The drawing under review shows one solid part. Ordinate dimensions are in mm from its lowest x, y, z. Round coordinates to 2 decimals unless told otherwise and drop trailing zeros. Order: outer loops, then holes, each group sorted by start corner. A loop starts at its lowest first (then second) coordinate and runs counter-clockwise, first axis right, second up.
1) Consider section C-C (z = 1.75). Give the boundary of the cut face in (x, y).
2) Consider section B-B (y = 25). Give the boundary of the cut face in (x, z), then the cut area to 3 significant figures.
3) To check wall thickness, follow L1, parallel to Y at x = 16, z = 3; L2, parallel to Y at x = 19.5, z = 6.75; L3, parallel to X at y = 59, z = 4.5. State the ranges of each line that lie inside material, in increasing order.
4) Clearance check with flat-ended pins moving along their axes: P1, Ø1, axis at x = 22.5, y = 40, coming from the -Z side; P2, Ø1.5, axis at x = 10, z = 5, coming from the -Y side. State where each tip first meets the part, or that it passes through.
5) Consider section A-A (x = 16). Give the boundary of the cut face in (y, z), then the cut area to 3 significant figures.
6) Mouldability with a two-part tool opening along Y and no side actions: class the marked faces 1, 2 and 3 as pulls with the +Y half, pulls with the -Y half, needs draft (parallel to the pull), parting line crosses it, or undercut.
7) Consider section D-D (y = 62). Give the boundary of the cut face in (x, z).
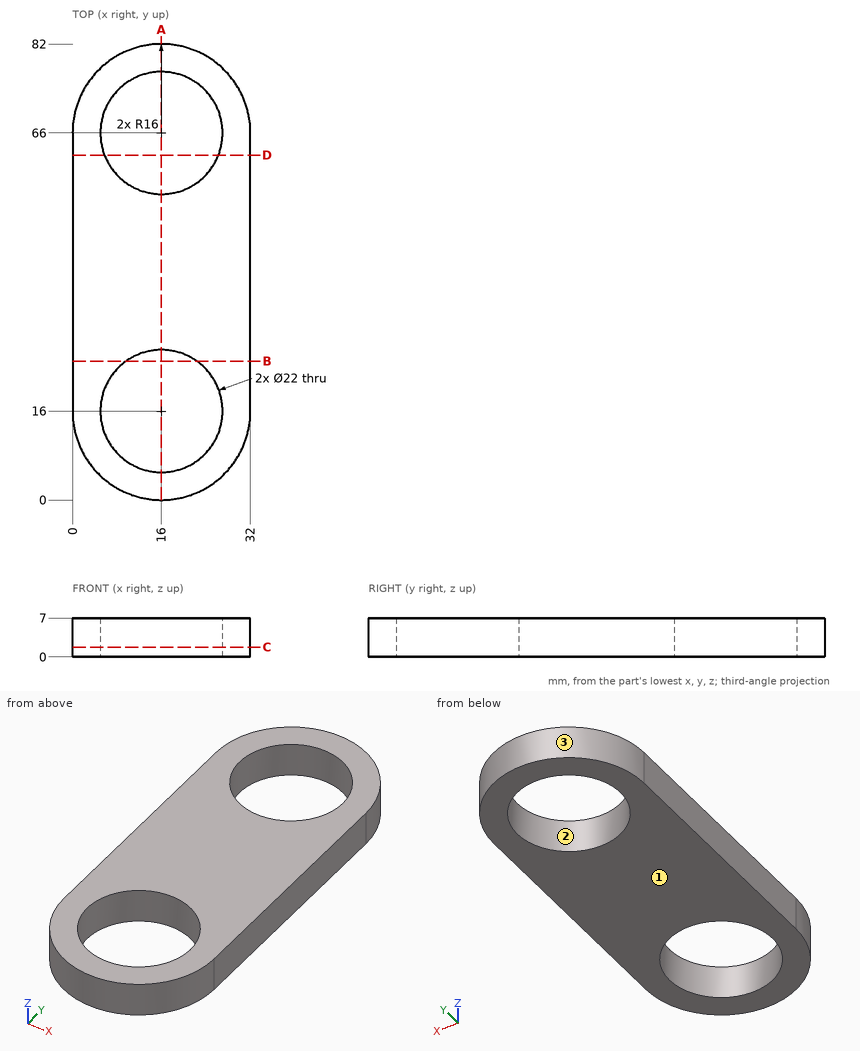
Answer below:
1. outline: (0, 16) arc R16 ccw to (32, 16) - (32, 66) arc R16 ccw to (0, 66) - close; hole circle Ø22 at (16, 16); hole circle Ø22 at (16, 66)
2. outline: (0, 0) - (9.68, 0) - (9.68, 7) - (0, 7) - close; (22.32, 0) - (32, 0) - (32, 7) - (22.32, 7) - close
2. area: 135 mm2
3. L1: y = 0 to 5, 27 to 55, 77 to 82
3. L2: y = 0.39 to 5.57, 26.43 to 55.57, 76.43 to 81.61
3. L3: x = 0 to 7.51, 24.49 to 32
4. P1: stops at z = 0
4. P2: stops at y = 0.89
5. outline: (0, 0) - (5, 0) - (5, 7) - (0, 7) - close; (27, 0) - (55, 0) - (55, 7) - (27, 7) - close; (77, 0) - (82, 0) - (82, 7) - (77, 7) - close
5. area: 266 mm2
6. face 1: needs draft
6. face 2: undercut
6. face 3: pulls with the +Y half
7. outline: (0, 0) - (5.75, 0) - (5.75, 7) - (0, 7) - close; (26.25, 0) - (32, 0) - (32, 7) - (26.25, 7) - close
